Can you work these out from the model? Positions are in its coordinate system, mm. Face numbers are marked on the shaded views. A direction names the side the tool comes from. Give positions to 0.01 mm unless a question says otherwise; leave off trailing zeros. Loops run counter-clockwise (first coordinate to the right, second up) from the corner with the lowest first, then second, coordinate; pieces in that order, holes last. Notation, with made-up numbers: M 52,85 L 97,85 A15 cw 97,94 Z; hole C 13,46.5 d11. An arc over 180 degrees is marked long. Answer as a JSON object with one key per item and string values.
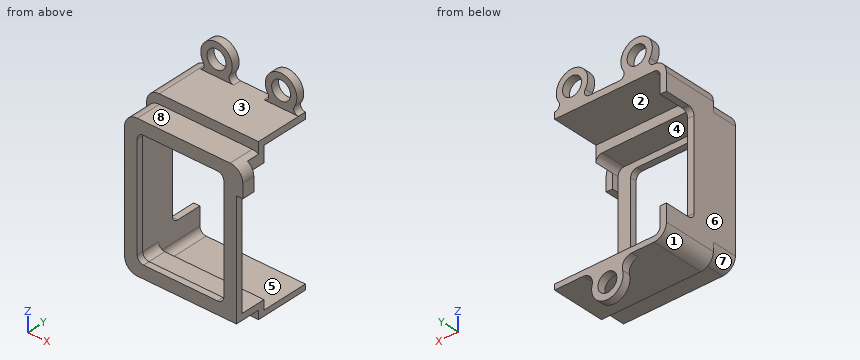
Autodesk Inventor part; units mm, degrees
ref_plane "Work Plane1" through (0, 8, 0) normal (0, 1, 0) x (1, 0, 0)
ref_plane "YZ Plane" through (0, 0, 0) normal (1, 0, 0) x (0, 1, 0)
ref_plane "XZ Plane" through (0, 0, 0) normal (0, 1, 0) x (-1, 0, 0)
sketch "Sketch1" plane through (0, 0, 0) normal (0, 1, 0) x (-1, 0, 0)
  arc A0 (31.569, 13.7227) -> (30.069, 12.2227) centre (31.569, 12.2227) ccw
  line L0 (31.569, 13.7227) -> (34.069, 13.7227)
  line L1 (34.069, 13.7227) -> (34.069, 18.9227)
  line L2 (32.069, 20.9227) -> (2.569, 20.9227)
  line L3 (34.069, -13.2773) -> (31.569, -13.2773)
  arc A1 (30.069, -11.7773) -> (31.569, -13.2773) centre (31.569, -11.7773) ccw
  arc A2 (34.069, 18.9227) -> (32.069, 20.9227) centre (32.069, 18.9227) ccw
  arc A3 (34.0195, 22.4149) -> (32.069, 23.9727) centre (32.069, 21.9727) ccw
  line L4 (32.069, 23.9727) -> (-23.931, 23.9727)
  arc A4 (-23.931, 23.9727) -> (-25.931, 21.9727) centre (-23.931, 21.9727) ccw
  line L5 (-25.931, 21.9727) -> (-25.931, -21.0273)
  arc A5 (-25.931, -21.0273) -> (-23.931, -23.0273) centre (-23.931, -21.0273) ccw
  line L6 (-23.931, -23.0273) -> (32.069, -23.0273)
  arc A6 (32.069, -23.0273) -> (33.899, -21.8341) centre (32.069, -21.0273) ccw
  arc A7 (32.069, -20.2773) -> (34.069, -18.2773) centre (32.069, -18.2773) ccw
  line L7 (32.069, -20.2773) -> (0.569, -20.2773)
  line L8 (34.069, -13.2773) -> (34.069, 13.7227)
  line L9 (0.569, -22.2773) -> (0.569, 18.9227)
  line L10 (30.069, -11.7773) -> (30.069, 12.2227)
  line L11 (34.069, -18.2773) -> (34.069, -13.2773)
  line L12 (2.569, 22.9227) -> (32.069, 22.9227)
  line L13 (0.569, -22.2773) -> (32.069, -22.2773)
  arc A8 (32.069, -22.2773) -> (36.069, -18.2773) centre (32.069, -18.2773) ccw
  line L14 (36.069, -18.2773) -> (36.069, 18.9227)
  arc A9 (2.569, 20.9227) -> (0.569, 18.9227) centre (2.569, 18.9227) ccw
  line L15 (-1.431, 14.4227) -> (-1.431, 18.9227)
  arc A10 (2.569, 22.9227) -> (-1.431, 18.9227) centre (2.569, 18.9227) ccw
  arc A11 (36.069, 18.9227) -> (32.069, 22.9227) centre (32.069, 18.9227) ccw
  line L16 (-1.431, 14.4227) -> (0.569, 14.4227)
  point P0 (0.569, 20.9227)
  dimension "d8" = 2
  dimension "d9" = 2
  dimension "d66" = 2
  dimension "d67" = 2
  dimension "d68" = 4.5
  dimension "d69" = 4
extrude "Extrusion3" add sketch "Sketch1" against normal blind 2 contours L0 L8 L3 A1 L10 A0 | A0 L10 A1 L3 L11 A7 L7 L9 A9 L2 A2 L1 L0 | L1 A2 L2 A9 L9 L16 L15 A10 L12 A11 L14 A8 L13 L7 A7 L11 L8
ref_plane "Work Plane1" through (0, 8, 0) normal (0, 1, 0) x (1, 0, 0)
extrude "Extrusion4" add sketch "Sketch1" along normal blind 8 contours L1 A2 L2 A9 L9 L16 L15 A10 L12 A11 L14 A8 L13 L7 A7 L11 L8
sketch "Sketch2" plane through (0, 8, 0) normal (0, 1, 0) x (1, 0, 0)
  line L0 (-0.569, 22.2773) -> (-0.569, 22.2773)
  line L1 (-0.569, 22.2773) -> (-0.569, 22.2773)
  line L2 (-36.069, -21.9727) -> (-36.069, 21.0273)
  line L3 (-32.069, -25.9727) -> (-0.569, -25.9727)
  line L4 (-0.569, -14.4227) -> (-0.569, -18.9227)
  line L5 (-0.569, -25.9727) -> (-0.569, -18.9227)
  line L6 (-0.569, -14.4227) -> (-0.569, 20.2773)
  line L7 (-0.569, 25.0273) -> (-32.069, 25.0273)
  line L8 (-0.569, 23.2773) -> (-32.069, 23.2773)
  line L9 (-32.069, 22.2773) -> (-0.569, 22.2773)
  arc A0 (-36.069, -21.9727) -> (-32.069, -25.9727) centre (-32.069, -21.9727) ccw
  line L10 (-0.569, -23.9227) -> (-32.069, -23.9227)
  line L11 (-34.069, -21.9227) -> (-34.069, 21.2773)
  line L12 (-34.069, 18.2773) -> (-34.069, -18.9227)
  arc A1 (-32.069, 23.2773) -> (-34.069, 21.2773) centre (-32.069, 21.2773) ccw
  arc A2 (-32.069, 25.0273) -> (-36.069, 21.0273) centre (-32.069, 21.0273) ccw
  arc A3 (-34.069, -21.9227) -> (-32.069, -23.9227) centre (-32.069, -21.9227) ccw
  line L13 (-34.069, -18.9227) -> (-34.069, 18.2773)
  line L14 (-36.069, 18.2773) -> (-36.069, -18.9227)
  line L15 (-32.069, 20.2773) -> (-0.569, 20.2773)
  line L16 (-2.569, -20.9227) -> (-32.069, -20.9227)
  line L17 (-32.069, -22.9227) -> (-2.569, -22.9227)
  line L18 (-0.569, 25.0273) -> (-0.569, 22.2773)
  line L19 (-0.569, 20.2773) -> (-0.569, 22.2773)
  line L20 (-0.569, 20.2773) -> (-32.069, 20.2773)
  arc A4 (-32.069, 20.2773) -> (-34.069, 18.2773) centre (-32.069, 18.2773) ccw
  line L21 (-34.069, 18.2773) -> (-34.069, -18.9227)
  arc A5 (-34.069, -18.9227) -> (-32.069, -20.9227) centre (-32.069, -18.9227) ccw
  line L22 (-32.069, -20.9227) -> (-2.569, -20.9227)
  arc A6 (-2.569, -20.9227) -> (-0.569, -18.9227) centre (-2.569, -18.9227) ccw
  line L23 (-0.569, -18.9227) -> (-0.569, -14.4227)
  line L24 (-0.569, -14.4227) -> (-0.569, 20.2773)
  dimension "d79" = 43
  dimension "d80" = 31.5
  dimension "d81" = 4
  dimension "d83" = 4.75
  dimension "d85" = 1
  dimension "d87" = 1
extrude "Extrusion7" add sketch "Sketch2" against normal blind 2 contours L2 A2 L7 L18 L8 A1 L11 A3 L10 L5 L3 A0 | L10 A3 L11 A5 L16 A6 L5 | L18 L19 L15 A4 L11 A1 L8
extrude "Extrusion8" add sketch "Sketch2" along normal blind 15 contours L2 A2 L7 L18 L8 A1 L11 A3 L10 L5 L3 A0
sketch "Sketch5" plane through (0, 23, 0) normal (0, 1, 0) x (1, 0, 0)
  circle A0 centre (-17.319, 30.0273) radius 5
  circle A1 centre (-17.319, 30.0273) radius 3
  arc A2 (-12.4777, 28.7773) -> (-9.573, 25.0273) centre (-9.573, 28.0273) ccw
  arc A3 (-25.0649, 25.0273) -> (-22.1602, 28.7773) centre (-25.0649, 28.0273) ccw
  circle A4 centre (-6.0917, -30.9727) radius 5
  circle A5 centre (-6.0917, -30.9727) radius 3
  arc A6 (-10.305, -28.2804) -> (-11.569, -25.9727) centre (-11.569, -27.4727) ccw
  arc A7 (-0.6145, -25.9727) -> (-1.8785, -28.2804) centre (-0.6145, -27.4727) ccw
  circle A8 centre (-26.5917, -30.9727) radius 5
  circle A9 centre (-26.5917, -30.9727) radius 3
  arc A10 (-21.1145, -25.9727) -> (-22.3785, -28.2804) centre (-21.1145, -27.4727) ccw
  line L0 (-11.569, -25.9727) -> (-0.6145, -25.9727)
  arc A11 (-30.805, -28.2804) -> (-32.069, -25.9727) centre (-32.069, -27.4727) ccw
  line L1 (-32.069, -25.9727) -> (-0.569, -25.9727)
  arc A12 (-36.069, -21.9727) -> (-32.069, -25.9727) centre (-32.069, -21.9727) ccw
  line L2 (-0.569, -22.3868) -> (-0.569, -25.9727)
  line L3 (-32.069, -25.9727) -> (-0.569, -25.9727)
  line L4 (-0.569, 25.0273) -> (-32.069, 25.0273)
  line L5 (-36.069, 21.0273) -> (-36.069, -21.9727)
  point P0 (0, 0)
  point P1 (-6.0917, -25.9727)
  point P2 (-26.5917, -25.9727)
  dimension "d34" = 10
  dimension "d35" = 6
  dimension "d38" = 3
  dimension "d39" = 3
  dimension "d40" = 10
  dimension "d41" = 6
  dimension "d42" = 3
  dimension "d43" = 3
  dimension "d44" = 10
  dimension "d45" = 6
  dimension "d47" = 3
  dimension "d49" = 20.5
  dimension "d88" = 3
  dimension "d89" = 18.75
extrude "Extrusion10" add sketch "Sketch5" against normal blind 2.5
sketch "Sketch6" plane through (0, -2, 0) normal (0, -1, 0) x (1, 0, 0)
  line L0 (-0.569, -22.2773) -> (-0.569, 14.4227)
  line L1 (-2.569, 22.9227) -> (-32.069, 22.9227)
  arc A0 (-32.069, 22.9227) -> (-36.069, 18.9227) centre (-32.069, 18.9227) ccw
  line L2 (-36.069, 18.9227) -> (-36.069, -18.2773)
  arc A1 (-36.069, -18.2773) -> (-32.069, -22.2773) centre (-32.069, -18.2773) ccw
  line L3 (-32.069, -22.2773) -> (-0.569, -22.2773)
  line L4 (-30.069, 18.9227) -> (-6.569, 18.9227)
  line L5 (-4.569, 16.9227) -> (-4.569, -16.2773)
  line L6 (-6.569, -18.2773) -> (-30.069, -18.2773)
  line L7 (-32.069, -16.2773) -> (-32.069, 16.9227)
  arc A2 (-6.569, -18.2773) -> (-4.569, -16.2773) centre (-6.569, -16.2773) ccw
  arc A3 (-32.069, -16.2773) -> (-30.069, -18.2773) centre (-30.069, -16.2773) ccw
  arc A4 (-30.069, 18.9227) -> (-32.069, 16.9227) centre (-30.069, 16.9227) ccw
  arc A5 (-4.569, 16.9227) -> (-6.569, 18.9227) centre (-6.569, 16.9227) ccw
  line L8 (-0.569, 14.4227) -> (1.431, 14.4227)
  line L9 (1.431, 14.4227) -> (1.431, 18.9227)
  arc A6 (1.431, 18.9227) -> (-2.569, 22.9227) centre (-2.569, 18.9227) ccw
  point P0 (0, 0)
  point P1 (-4.569, 18.9227)
  point P2 (-4.569, -18.2773)
  dimension "d52" = 4
  dimension "d53" = 37.2
  dimension "d54" = 27.5
  dimension "d55" = 4
  dimension "d56" = 2
extrude "Extrusion11" cut sketch "Sketch6" against normal blind 2 contours L4 A5 L5 A2 L6 A3 L7 A4
sketch "Sketch7" plane through (-36.069, -2, -18.2773) normal (-1, 0, 0) x (0, 0, 1)
  line L0 (2.75, 25) -> (34.75, 25)
  line L1 (34.75, 25) -> (34.75, 17)
  line L2 (32.75, 15) -> (4.75, 15)
  line L3 (2.75, 17) -> (2.75, 25)
  arc A0 (2.75, 17) -> (4.75, 15) centre (4.75, 17) ccw
  arc A1 (32.75, 15) -> (34.75, 17) centre (32.75, 17) ccw
  line L4 (40.25, 8) -> (40.25, 25)
  line L5 (-2.75, 25) -> (40.25, 25)
  point P0 (18.2773, 2)
  point P1 (34.75, 21)
  dimension "d59" = 2
  dimension "d61" = 32
  dimension "d90" = 5.5
  dimension "d91" = 10
extrude "Extrusion12" cut sketch "Sketch7" against normal blind 6
sketch "Sketch8" plane through (0, 8, 0) normal (0, 1, 0) x (1, 0, 0)
  line L0 (-0.569, -14.4227) -> (-0.569, -18.9227)
  line L1 (1.431, -14.4227) -> (-0.569, -14.4227)
  line L2 (1.431, -18.9227) -> (1.431, -14.4227)
  arc A0 (-0.569, -22.3868) -> (1.431, -18.9227) centre (-2.569, -18.9227) ccw
  line L3 (-0.569, -23.9727) -> (-0.569, -18.9227)
  point P0 (0, 0)
  point P1 (-0.4025, -22.2852)
  point P2 (-0.4025, -22.2852)
  point P3 (-2.569, -22.9227)
  point P4 (-0.569, -22.3868)
extrude "Extrusion13" cut sketch "Sketch8" against normal blind 6
equation "\"shrink\" = 0.25"
properties part number "CO-1-06-motorControllersMount"
1) For the marked faces 4, 5, 6, 7 and 8, which set-ups out of +Z, -Z, +X, -X, +Y, -Y let a thin tool reach every point of the face, with its end or its side?
Answer list:
{"face 4": "+Y", "face 5": "+X, +Y", "face 6": "+Z, -Z, -X, +Y, -Y", "face 7": "-Z, -X, -Y", "face 8": "+Z, +X, -X, -Y"}
2) Suppose I cut it at A-A, the plane y = 18.25. Write out the boundary of the cut face in (x, z), and give its area (3 significant figures).
Answer list:
{"outline": "M -36.07,-21.03 A4 ccw -32.07,-25.03 L -0.57,-25.03 L -0.57,-23.28 L -32.07,-23.28 A2 cw -34.07,-21.28 L -34.07,-15.53 L -36.07,-15.53 Z; M -36.07,16.47 L -34.07,16.47 L -34.07,21.92 A2 cw -32.07,23.92 L -0.57,23.92 L -0.57,25.97 L -32.07,25.97 A4 ccw -36.07,21.97 Z", "area": "160 mm^2"}
3) Please list where these lines run through material, in increasing order: line 1 along Z through (x, y) = (-2.5, 13.75); line 2 along Z through (x, y) = (-22.5, 2); line 3 along X through (y, z) = (-0.75, -8). Write a range as from..to.
Answer list:
{"line 1": "-25.03..-23.28, 23.92..25.97", "line 2": "-22.28..-20.28, 20.92..22.92", "line 3": "-36.07..-32.07, -4.57..-0.57"}
4) Will these pins go through, and if not, where does the flat tip stop? pin 1 Ø4.5 at (x, y) = (-22.5, 16) entering from +Z; pin 2 Ø8 at (x, y) = (-14.5, 7.5) entering from -Z; pin 3 Ø5 at (y, z) = (14, -25.5) entering from +X.
Answer list:
{"pin 1": "z = 25.97", "pin 2": "z = -25.03", "pin 3": "x = -0.57"}
5) Suppose I cut it at B-B, the plane z = 6. Write out the boundary of the cut face in (x, y).
Answer list:
{"outline": "M -36.07,-2 L -32.07,-2 L -32.07,0 L -34.07,0 L -34.07,13 L -36.07,13 Z; M -4.57,-2 L -0.57,-2 L -0.57,0 L -4.57,0 Z"}
6) Suppose I cut it at C-C, the plane x = -16. Write out the boundary of the cut face in (y, z).
Answer list:
{"outline": "M -2,-22.28 L 6,-22.28 L 6,-25.03 L 20.5,-25.03 L 20.5,-27.33 L 23,-27.33 L 23,-23.28 L 8,-23.28 L 8,-20.28 L 0,-20.28 L 0,-18.28 L -2,-18.28 Z; M -2,18.92 L 0,18.92 L 0,20.92 L 8,20.92 L 8,23.92 L 23,23.92 L 23,25.97 L 6,25.97 L 6,22.92 L -2,22.92 Z; M 20.5,-34.85 L 23,-34.85 L 23,-32.72 L 20.5,-32.72 Z"}
7) Suppose I cut it at D-D, the plane y = 7. Write out the boundary of the cut face in (x, z).
Answer list:
{"outline": "M -36.07,-21.03 A4 ccw -32.07,-25.03 L -0.57,-25.03 L -0.57,-20.28 L -32.07,-20.28 A2 cw -34.07,-18.28 L -34.07,18.92 A2 cw -32.07,20.92 L -2.57,20.92 A2 cw -0.57,18.92 L -0.57,25.97 L -32.07,25.97 A4 ccw -36.07,21.97 Z"}
8) If we mould it in two halves opening along Z, with no side actions, what happens to the marked faces 1, 2 and 3? For each: +Z half, -Z half, draft (parallel to the pull), parting line (faces both ways), or undercut.
Answer list:
{"face 1": "-Z half", "face 2": "undercut", "face 3": "+Z half"}
